For this review, take the finished solid that the model builds, in its own axes (mm). Face numbers are marked on the shaded views. A direction names the side the tool comes from. Coordinates: 2 decimals unless noted, no trailing zeros. Loops run counter-clockwise (first coordinate to the right, second up) from the corner with the lowest first, then second, coordinate; pieces in that order, holes last. Notation, with made-up numbers: (70, 68) -> (81, 68) arc R17 ccw to (81, 73) -> close; hole circle Ø9 at (33, 61). An arc over 180 degrees is marked (long way). Answer in a Markdown table with one row per item.
from build123d import *

# Parameters (mm, degrees)
SKETCH1_R               = 2.485
SKETCH1_W               = 55.97
SKETCH1_H               = 4
SKETCH1_W_2             = 2
BOSS_EXTRUDE1_DEPTH     = 6
SKETCH2_R               = 2.485
BOSS_EXTRUDE2_DEPTH     = 2
BOSS_EXTRUDE3_DEPTH     = 20.015
SKETCH6_R               = 2.485
CUT_EXTRUDE3_DEPTH      = 10
SKETCH11_R              = 17.715
BOSS_EXTRUDE4_DEPTH     = 8
BOSS_EXTRUDE5_START     = 20
SKETCH11_3_R            = 17.715
SKETCH11_3_R_2          = 12.715
BOSS_EXTRUDE5_DEPTH     = 20
BOSS_EXTRUDE7_DEPTH     = 20
CUT_EXTRUDE7_DEPTH      = 63.485922014
CUT_EXTRUDE7_DEPTH_BACK = 63.485922014
CUT_EXTRUDE8_DEPTH      = 72.185604057
CUT_EXTRUDE8_DEPTH_BACK = 72.185604057
FILLET1_R               = 2.5
CUT_EXTRUDE9_DEPTH      = 59.876909311
CUT_EXTRUDE9_DEPTH_BACK = 59.876909311
SKETCH16_R              = 2.6
SKETCH17_R              = 5.436873337
SKETCH17_R_2            = 2.6
CUT_EXTRUDE10_DEPTH     = 12
BOSS_EXTRUDE8_REACH     = 72.478
SKETCH18_R              = 5.436873337
CHAMFER1_SIZE           = 8
CHAMFER2_SIZE           = 8


# Some blends are built 0.0001 mm under size
with BuildPart() as part:
    # Sketch1 → Boss-Extrude1 (new, symmetric)
    # profile 1 of 8: a face of its own
    with BuildSketch(Plane(origin=(0, 0, 0), x_dir=(1, 0, 0), z_dir=(0, 1, 0))):
        with BuildLine():
            ThreePointArc((24, -0.115), (21.182179477, -1.282179477), (20.015, -4.1))
            Line((20.015, -4.1), (20.015, -10.015))
            Line((20.015, -10.015), (-20.015, -10.015))
            Line((-20.015, -10.015), (-20.015, 10.015))
            Line((-20.015, 10.015), (20.015, 10.015))
            Line((20.015, 10.015), (20.015, 4.1))
            ThreePointArc((20.015, 4.1), (21.182179477, 1.282179477), (24, 0.115))
            ThreePointArc((24, 0.115), (26.817820523, 1.282179477), (27.985, 4.1))
            Line((27.985, 4.1), (27.985, 14.015))
            Line((27.985, 14.015), (-27.985, 14.015))
            Line((-27.985, 14.015), (-27.985, -14.015))
            Line((-27.985, -14.015), (27.985, -14.015))
            Line((27.985, -14.015), (27.985, -4.1))
            ThreePointArc((27.985, -4.1), (26.817820523, -1.282179477), (24, -0.115))
        make_face()
        with Locations(Location((-24, -5, 0), (0, 0, 270))):
            Circle(SKETCH1_R, mode=Mode.SUBTRACT)
        with Locations(Location((-24, 5, 0), (0, 0, 270))):
            Circle(SKETCH1_R, mode=Mode.SUBTRACT)
        with Locations(Location((24, -5, 0), (0, 0, 270))):
            Circle(SKETCH1_R, mode=Mode.SUBTRACT)
        with Locations(Location((24, 5, 0), (0, 0, 270))):
            Circle(SKETCH1_R, mode=Mode.SUBTRACT)
    # profile 2 of 8: a face of its own
    with BuildSketch(Plane(origin=(0, 0, 0), x_dir=(1, 0, 0), z_dir=(0, 1, 0))):
        with Locations((0, -16.015)):
            Rectangle(SKETCH1_W, SKETCH1_H)
    # profile 3 of 8: a face of its own
    with BuildSketch(Plane(origin=(0, 0, 0), x_dir=(1, 0, 0), z_dir=(0, 1, 0))):
        Polygon((27.985, 4.1), (27.985, 0.115), (29.985, 0.115), (29.985, 14.015), (27.985, 14.015), align=None)
    # profile 4 of 8: a face of its own
    with BuildSketch(Plane(origin=(0, 0, 0), x_dir=(1, 0, 0), z_dir=(0, 1, 0))):
        Polygon((29.985, -0.115), (27.985, -0.115), (27.985, -4.1), (27.985, -14.015), (29.985, -14.015), align=None)
    # profile 5 of 8: a face of its own
    with BuildSketch(Plane(origin=(0, 0, 0), x_dir=(1, 0, 0), z_dir=(0, 1, 0))):
        with BuildLine():
            Line((27.985, -4.1), (27.985, -0.115))
            Line((27.985, -0.115), (24, -0.115))
            ThreePointArc((24, -0.115), (26.817820523, -1.282179477), (27.985, -4.1))
        make_face()
    # profile 6 of 8: a face of its own
    with BuildSketch(Plane(origin=(0, 0, 0), x_dir=(1, 0, 0), z_dir=(0, 1, 0))):
        with BuildLine():
            Line((24, 0.115), (27.985, 0.115))
            Line((27.985, 0.115), (27.985, 4.1))
            ThreePointArc((27.985, 4.1), (26.817820523, 1.282179477), (24, 0.115))
        make_face()
    # profile 7 of 8: a face of its own
    with BuildSketch(Plane(origin=(0, 0, 0), x_dir=(1, 0, 0), z_dir=(0, 1, 0))):
        with Locations((28.985, -16.015)):
            Rectangle(SKETCH1_W_2, SKETCH1_H)
    # profile 8 of 8: a face of its own
    with BuildSketch(Plane(origin=(0, 0, 0), x_dir=(1, 0, 0), z_dir=(0, 1, 0))):
        Polygon((-29.985, 14.015), (-29.985, -18.015), (-27.985, -18.015), (-27.985, -14.015), (-27.985, 14.015), align=None)
    extrude(amount=BOSS_EXTRUDE1_DEPTH, both=True)

    # Sketch2 → Boss-Extrude2 (add)
    with BuildSketch(Plane.XZ.offset(6)):
        with Locations(Location((24, -5, 0), (0, 0, 90))):
            Circle(SKETCH2_R)
        with Locations(Location((24, 5, 0), (0, 0, 90))):
            Circle(SKETCH2_R)
        with Locations(Location((-24, -5, 0), (0, 0, 90))):
            Circle(SKETCH2_R)
        with Locations(Location((-24, 5, 0), (0, 0, 90))):
            Circle(SKETCH2_R)
    extrude(amount=-BOSS_EXTRUDE2_DEPTH)

    # Sketch5 → Boss-Extrude3 (add)
    with BuildSketch(Plane(origin=(0, 0, 0), x_dir=(0, 0, -1), z_dir=(1, 0, 0))):
        Polygon((-18.015, -6), (-10.015, -6), (-10.015, -21.5), (6.985, -21.5), (6.985, -33.5), (-18.015, -33.5), align=None)
    extrude(amount=BOSS_EXTRUDE3_DEPTH)

    # Sketch6 → Cut-Extrude3 (cut)
    with BuildSketch(Plane.XZ.offset(33.5)):
        with Locations(Location((10.015, 0, 0), (0, 0, 270))):
            Circle(SKETCH6_R)
    extrude(amount=-CUT_EXTRUDE3_DEPTH, mode=Mode.SUBTRACT)

    # Sketch11 → Boss-Extrude4 (add)
    with BuildSketch(Plane.XY.offset(18.015)):
        with Locations((10.0075, 0)):
            Circle(SKETCH11_R)
    extrude(amount=-BOSS_EXTRUDE4_DEPTH)

    # Sketch11<3> → Boss-Extrude5 (add)
    with BuildSketch(Plane.XY.offset(18.015).offset(BOSS_EXTRUDE5_START)):
        with Locations((10.0075, 0)):
            Circle(SKETCH11_3_R)
        with Locations((10.0075, 0)):
            Circle(SKETCH11_3_R_2, mode=Mode.SUBTRACT)
    extrude(amount=-BOSS_EXTRUDE5_DEPTH)

    # Sketch13 → Boss-Extrude7 (add)
    with BuildSketch(Plane.XY.offset(38.015)):
        with BuildLine():
            ThreePointArc((20.015, -14.617495297), (10.0075, -17.715), (0, -14.617495297))
            Line((0, -14.617495297), (0, -33.5))
            Line((0, -33.5), (20.015, -33.5))
            Line((20.015, -33.5), (20.015, -14.617495297))
        make_face()
        with BuildLine():
            Line((-29.985, -6), (-6.660470032, -6))
            ThreePointArc((-6.660470032, -6), (-7.7075, 0), (-6.660470032, 6))
            Line((-6.660470032, 6), (-29.985, 6))
            Line((-29.985, 6), (-29.985, -6))
        make_face()
        with BuildLine():
            ThreePointArc((27.7225, 0), (27.458779525, -3.045335439), (26.675470032, -6))
            Line((26.675470032, -6), (29.985, -6))
            Line((29.985, -6), (29.985, 6))
            Line((29.985, 6), (26.675470032, 6))
            ThreePointArc((26.675470032, 6), (27.458779525, 3.045335439), (27.7225, 0))
        make_face()
    extrude(amount=-BOSS_EXTRUDE7_DEPTH)

    # Sketch14 → Cut-Extrude7 (cut, two sides: drawn at the far end of the back side and taken through both)
    with BuildSketch(Plane(origin=(0, 6, 0), x_dir=(1, 0, 0), z_dir=(0, 1, 0)).offset(-CUT_EXTRUDE7_DEPTH_BACK)):
        Polygon((-29.985, -38.015), (-6.660470032, -38.015), (-29.985, -14.690470032), align=None)
    extrude(amount=CUT_EXTRUDE7_DEPTH + CUT_EXTRUDE7_DEPTH_BACK, mode=Mode.SUBTRACT)

    # Sketch15 → Cut-Extrude8 (cut, two sides: drawn at the far end of the back side and taken through both)
    with BuildSketch(Plane(origin=(20.015, 0, 0), x_dir=(0, 0, -1), z_dir=(1, 0, 0)).offset(-CUT_EXTRUDE8_DEPTH_BACK)):
        Polygon((-19.132495297, -33.5), (-38.015, -14.617495297), (-38.015, -33.5), align=None)
    extrude(amount=CUT_EXTRUDE8_DEPTH + CUT_EXTRUDE8_DEPTH_BACK, mode=Mode.SUBTRACT)

    # Fillet1
    fillet1_edges = [part.edges().sort_by_distance(p)[0] for p in [
        (-29.985, 0, -14.015),
        (29.985, 0, -14.015),
    ]]
    fillet(fillet1_edges, radius=FILLET1_R)

    # Sketch16 → Cut-Extrude9 (cut, two sides: drawn at the far end of the back side and taken through both)
    with BuildSketch(Plane(origin=(0, 0, 0), x_dir=(1, 0, 0), z_dir=(0, 1, 0)).offset(-CUT_EXTRUDE9_DEPTH_BACK)):
        with Locations(Location((10.0075, -28.015, 0), (0, 0, 270))):
            Circle(SKETCH16_R)
    extrude(amount=CUT_EXTRUDE9_DEPTH + CUT_EXTRUDE9_DEPTH_BACK, mode=Mode.SUBTRACT)

    # Sketch17 → Cut-Extrude10 (cut)
    with BuildSketch(Plane.XZ.offset(33.5)):
        with Locations((10.0075, 28.015)):
            Circle(SKETCH17_R)
        with Locations(Location((10.0075, 28.015, 0), (0, 0, 90))):
            Circle(SKETCH17_R_2, mode=Mode.SUBTRACT)
    extrude(amount=-CUT_EXTRUDE10_DEPTH, mode=Mode.SUBTRACT)

    # Sketch18 → Boss-Extrude8 (add, up to next)
    with BuildSketch(Plane.XZ.offset(33.5), mode=Mode.PRIVATE) as boss_extrude8_sk1:
        with BuildLine():
            Line((29.985, 38.015), (-6.660470032, 38.015))
            Line((-6.660470032, 38.015), (-29.985, 14.690470032))
            Line((-29.985, 14.690470032), (-29.985, -11.515))
            ThreePointArc((-29.985, -11.515), (-29.252766953, -13.282766953), (-27.485, -14.015))
            Line((-27.485, -14.015), (27.485, -14.015))
            ThreePointArc((27.485, -14.015), (29.252766953, -13.282766953), (29.985, -11.515))
            Line((29.985, -11.515), (29.985, -8.115))
            Line((29.985, -8.115), (20.015, -8.115))
            Line((20.015, -8.115), (20.015, -10.015))
            Line((20.015, -10.015), (-20.015, -10.015))
            Line((-20.015, -10.015), (-20.015, 10.015))
            Line((-20.015, 10.015), (0, 10.015))
            Line((0, 10.015), (0, 19.132495297))
            Line((0, 19.132495297), (20.015, 19.132495297))
            Line((20.015, 19.132495297), (20.015, 10.015))
            Line((20.015, 10.015), (20.015, 8.115))
            Line((20.015, 8.115), (29.985, 8.115))
            Line((29.985, 8.115), (29.985, 38.015))
        make_face()
        with Locations(Location((10.0075, 28.015, 0), (0, 0, 270))):
            Circle(SKETCH18_R, mode=Mode.SUBTRACT)
    boss_extrude8_tool1 = extrude(boss_extrude8_sk1.sketch, amount=-BOSS_EXTRUDE8_REACH, mode=Mode.PRIVATE) - part.part
    add(boss_extrude8_tool1.solids().sort_by_distance((-0.47266, -33.5, 14.933652))[0])

    # Chamfer1
    chamfer1_edges = [part.edges().sort_by_distance(p)[0] for p in [
        (25, -6, -8.115),
        (25, -6, 8.115),
    ]]
    chamfer(chamfer1_edges, length=CHAMFER1_SIZE - 0.0001)  # a hair under: the kernel refuses the full size

    # Chamfer2
    # the kernel refuses this chamfer: 8 mm, written as the material it takes off along each edge
    with BuildSketch(Plane(origin=(29.985, -33.5, 8.115), x_dir=(-0.9996219169112968, -0.027495876610586487, 0), z_dir=(0, 0, 1))) as chamfer2_piece_1:
        Polygon((CHAMFER2_SIZE * 0.999621916911, -CHAMFER2_SIZE * 0.0274958766106), (-CHAMFER2_SIZE * 0.0274958766106, -CHAMFER2_SIZE * 0.999621916911), (0, 0), align=None)
    extrude(amount=50.473463904, mode=Mode.SUBTRACT)
    with BuildSketch(Plane(origin=(50.558463904, -33.5, 38.015), x_dir=(0, -0.027495876610586487, -0.9996219169112968), z_dir=(-1, 0, 0))) as chamfer2_piece_2:
        Polygon((CHAMFER2_SIZE * 0.999621916911, -CHAMFER2_SIZE * 0.0274958766106), (-CHAMFER2_SIZE * 0.0274958766106, -CHAMFER2_SIZE * 0.999621916911), (0, 0), align=None)
    extrude(amount=77.79239784, mode=Mode.SUBTRACT)
    with BuildSketch(Plane(origin=(7.887165806, -33.5, 52.562635839), x_dir=(0.7068394360706746, -0.027495876610586497, -0.7068394360706723), z_dir=(-0.7071067811865466, 0, -0.7071067811865486))) as chamfer2_piece_3:
        Polygon((CHAMFER2_SIZE * 0.999621916911, -CHAMFER2_SIZE * 0.0274958766106), (-CHAMFER2_SIZE * 0.0274958766106, -CHAMFER2_SIZE * 0.999621916911), (0, 0), align=None)
    extrude(amount=74.132794424, mode=Mode.SUBTRACT)


solid = part.part
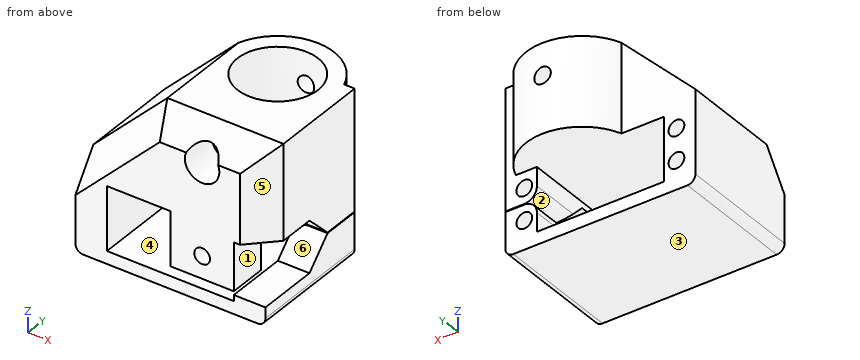
Item 1: For L1, parallel to X at y = 4, z = 5 (3 decimals); L2, parallel to Z at x = 10.5, y = -2 (3 decimals); L3, parallel to Z at x = -24, y = -1.5 (3 decimals), list the stretches that pass through material, from the lowest coordinate up.
Worked answers:
| item | result |
|---|---|
| L1 | -29.985 to -26.485, -21.515 to -20.015, 20.015 to 21.515, 26.485 to 29.985 |
| L2 | -14.015 to -10.015, 10.015 to 18.015 |
| L3 | -14.015 to -7.485, -2.515 to 2.515, 7.485 to 20.675 |
Item 2: Insertion check: pin 1 (3 mm diameter, centred on x = -18.5, y = -9.5, fed in from +Z); pin 2 (7 mm diameter, centred on x = 10, z = 27.5, fed in from -Y); pin 3 (3 mm diameter, centred on y = -28, z = 29, fed in from -X). Each pin has a flat end and moves straight along its axis. Give the tip position at first contact, or say it passes through.
Worked answers:
| item | result |
|---|---|
| pin 1 | z = 27.68 |
| pin 2 | y = -21.5 |
| pin 3 | x = -14.74 |
Item 3: The part is to be moulded in two halves that separate along X. For the marked faces 1, 2 and 3, say which applies: +X half, -X half, draft (parallel to the pull), parting line (faces both ways), or undercut.
Worked answers:
| item | result |
|---|---|
| face 1 | +X half |
| face 2 | undercut |
| face 3 | draft |
Item 4: Take a section at D-D, the plane x = 11. Count the separate pieces of the cut face and the enclosed holes in it, and give its area (3 significant figures).
Worked answers:
| item | result |
|---|---|
| separate pieces | 4 |
| enclosed holes | 0 |
| area | 1,020 mm² |
Item 5: Take a section at A-A, the plane y = 0. State the section outline as (x, z) points (1 decimal), and give its area (3 significant figures).
Worked answers:
| item | result |
|---|---|
| outline | (-30, -11.5) arc R2.5 ccw to (-27.5, -14) -> (27.5, -14) arc R2.5 ccw to (30, -11.5) -> (30, -0.1) -> (24, -0.1) arc R4 ccw to (20, -4.1) -> (20, -10) -> (-20, -10) -> (-20, 10) -> (20, 10) -> (20, 4.1) arc R4 ccw to (24, 0.1) -> (30, 0.1) -> (30, 38) -> (22.7, 38) -> (22.7, 18) -> (-2.7, 18) -> (-2.7, 38) -> (-6.7, 38) -> (-30, 14.7) -> close; hole circle Ø5 at (-24, -5); hole circle Ø5 at (-24, 5); hole circle Ø5 at (24, -5); hole circle Ø5 at (24, 5) |
| area | 1,450 mm² |
Item 6: For the marked faces 4, 5 and 6, list the 3-axis set-ups (+Z, -Z, +X, -X, +Y, -Y) from which the entire face can be reached by the end or side of a thin tool; tool diameter is ignored.
Worked answers:
| item | result |
|---|---|
| face 4 | +Y, -Y |
| face 5 | +Z, +X, -Y |
| face 6 | +X, -Y |
Item 7: Take a section at B-B, the plane x = 17. State the section outline as (y, z) points (3 decimals), and give its area (3 significant figures).
Worked answers:
| item | result |
|---|---|
| outline | (-33.5, -14.015) -> (6, -14.015) -> (6, -10.015) -> (-33.5, -10.015) -> close; (-33.5, -6.985) -> (-21.5, -6.985) -> (-21.5, 10.015) -> (16.277, 10.015) -> (16.277, 38.015) -> (10.62, 38.015) -> (10.62, 18.015) -> (-10.62, 18.015) -> (-10.62, 38.015) -> (-25.5, 38.015) -> (-33.5, 30.015) -> close |
| area | 1,300 mm² |
Item 8: Take a section at C-C, the plane z = 20. State the section outline as (x, y) points (1 decimal), and give its area (3 significant figures).
Worked answers:
| item | result |
|---|---|
| outline | (-24.7, -25.5) -> (-13.4, -33.5) -> (22, -33.5) -> (30, -25.5) -> (30, 6) -> (26.7, 6) arc R17.7 ccw to (-6.7, 6) -> (-24.7, 6) -> close; hole circle Ø25.4 at (10, 0) |
| area | 1,860 mm² |
